Verification items for this drawing (mm, ordinates from the low corner). A direction names the side the tool comes from. Coordinates: 2 decimals unless noted, no trailing zeros. Write each loop counter-clockwise with the first axis right and the second up, starting at its lowest first coordinate (ties: lowest second). Pieces come first, ordered by that corner, then holes. Notation, with made-up numbers: M -15,-23 L -5,-23 A35 ccw -5,16 Z; hole C -29.5,46.5 d3. An arc over 180 degrees is marked long. Answer as CSV lines item,"result". Start each with the question number.
1) Access from +Z, -Z, +X, -X, +Y, -Y to the whole of each face (thin tool, end or side, straight path). Record for the marked faces 4 and 5.
2) Material ranges on L1, parallel to Z at x = 6, y = 1.1; L2, parallel to Y at x = 6, z = 1.8; L3, parallel to Y at x = 6.75, z = 4, recorded low to high. Write a range as [from, to].
3) Draft check along X on the marked faces 1, 2 and 3. Enter one of: +X half, -X half, draft (parallel to the pull), parting line (faces both ways), or undercut.
4) Section check B-B (z = 5.75). Record the cut outline in (x, y), and give its area (3 significant figures).
5) Section check A-A (z = 3.25). Record the cut outline in (x, y), and give its area (3 significant figures).
6) Section check C-C (x = 6). State how many separate pieces and enclosed holes the cut face has, and give its area (3 significant figures).
7) Section check D-D (z = 2.5). Record the cut outline in (x, y), and give its area (3 significant figures).
8) Go/stop test with a flat-tipped pin: pin 1 Ø2 at (y, z) = (7.5, 0.5) entering from +X. Record where the tip stops, or that it passes through.
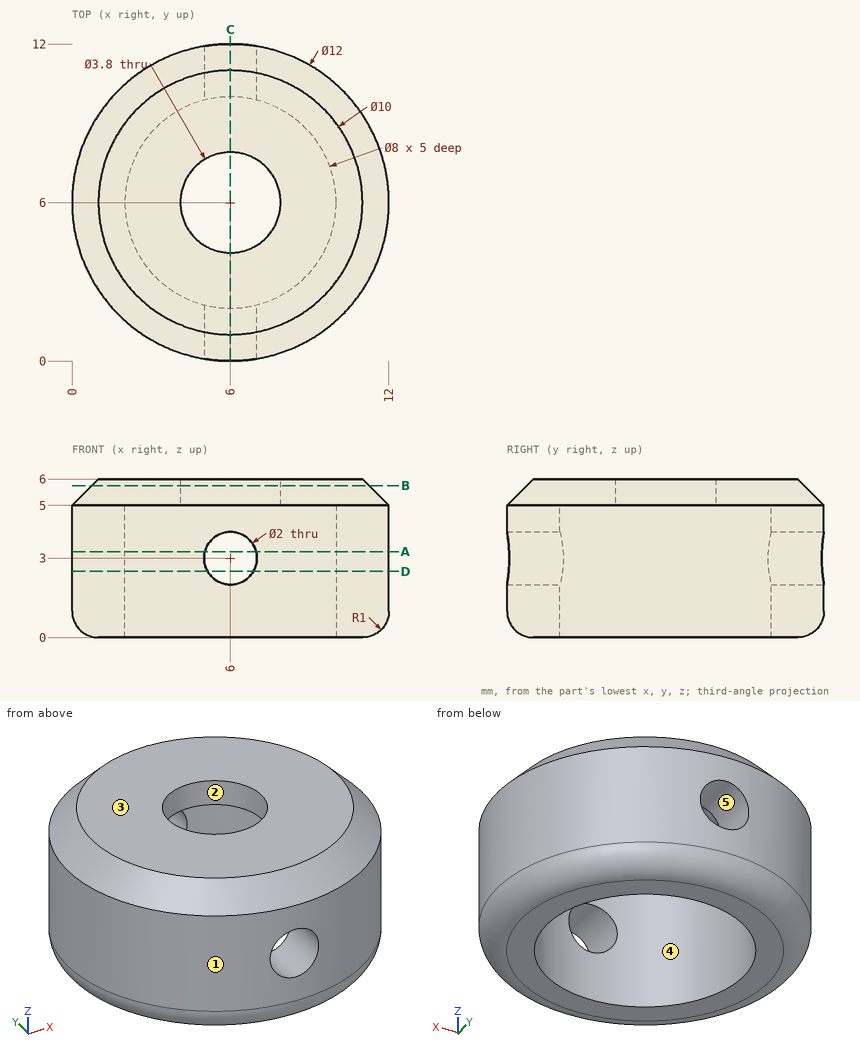
Results found:
1,face 4,"-Z"
1,face 5,"+Y, -Y"
2,L1,"z = [0, 2], [4, 6]"
2,L2,"y = [0, 2], [10, 12]"
2,L3,"y = [0.05, 2.07], [9.93, 11.95]"
3,face 1,"parting line"
3,face 2,"undercut"
3,face 3,"draft"
4,outline,"C 6,6 d10.5; hole C 6,6 d3.8"
4,area,"75.2 mm2"
5,outline,"M 5.03,0.08 L 5.03,2.12 A4 cw 5.03,9.88 L 5.03,11.92 A6 ccw Z; M 6.97,0.08 A6 ccw 6.97,11.92 L 6.97,9.88 A4 cw 6.97,2.12 Z"
5,area,"55.0 mm2"
6,separate pieces,"4"
6,enclosed holes,"0"
6,area,"18.8 mm2"
7,outline,"M 5.13,0.06 L 5.13,2.09 A4 cw 5.13,9.91 L 5.13,11.94 A6 ccw Z; M 6.87,0.06 A6 ccw 6.87,11.94 L 6.87,9.91 A4 cw 6.87,2.09 Z"
7,area,"55.9 mm2"
8,pin 1,"stops at x = 11.97"
